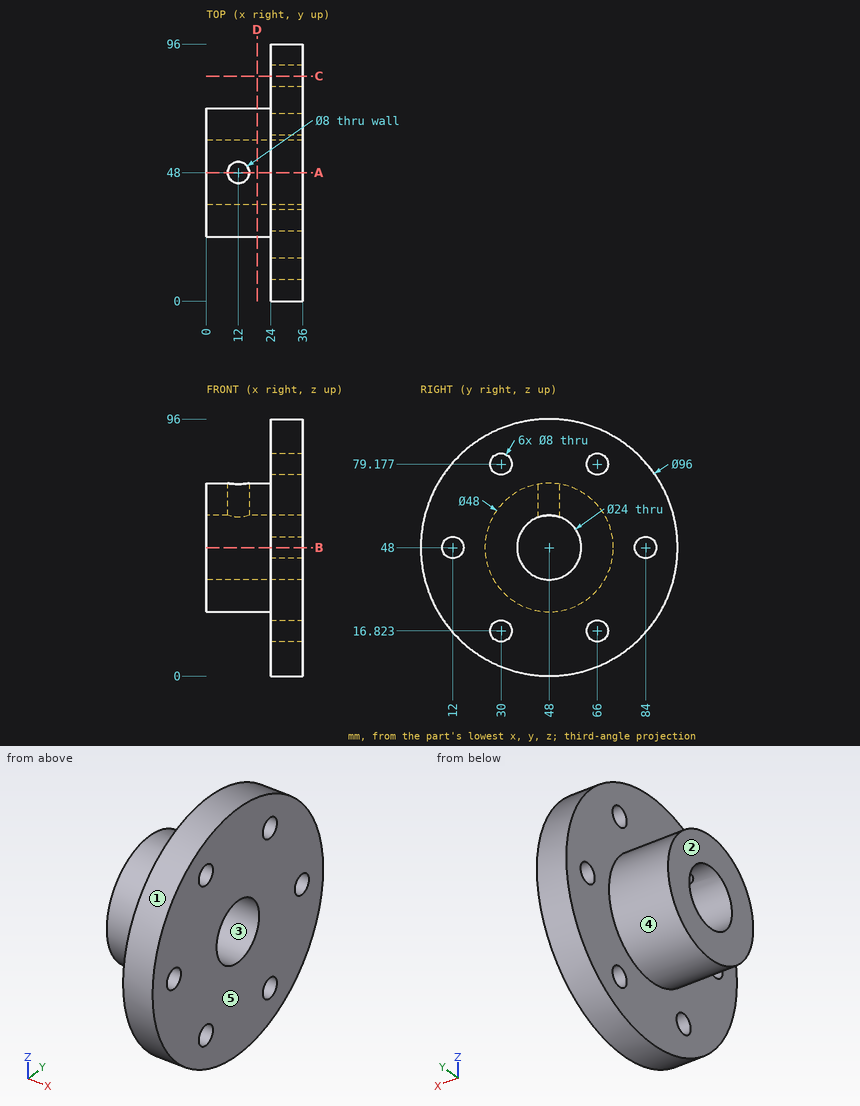
The figure shows three views and two pictorial views of one solid part (mm, origin at its lowest corner). Answer the questions. A direction names the side the tool comes from. Coordinates: 2 decimals unless noted, no trailing zeros. Loops run counter-clockwise (first coordinate to the right, second up) from the corner with the lowest first, then second, coordinate; pieces in that order, holes last. Notation, with made-up numbers: M 14.5,80 L 71.5,80 A18 ccw 71.5,115 Z; hole C 25.25,-14 d6. An arc over 180 degrees is marked long. Answer as CSV lines item,"result". Start each with the question number.
(1) For the marked faces 4 and 5, determine the directions among +Z, -Z, +X, -X, +Y, -Y from which every point of the face is accessible in a straight line to the end or side of a thin tool.
(2) The part is cut by section D-D (x = 19). Give the vertices of the cut face in (y, z), and give its area (3 significant figures).
(3) Given pin 1 (4 mm diameter, centred on x = 5.5, z = 59, fed in from -Y); pin 2 (1 mm diameter, centred on x = 12.5, z = 59, fed in from -Y); pin 3 (3 mm diameter, centred on y = 50, z = 15, fed in from -X), each flat-ended and moving along its own axis, determine where each tip first touches the part or whether it passes through.
(4) The part is cut by section B-B (z = 48). Give the vertices of the cut face in (x, y).
(5) The part is cut by section C-C (y = 84). Give the vertices of the cut face in (x, z).
(6) The mould has two halves that part along Z. Classify the marked faces 1, 2 and 3: pulls with the +Z half, pulls with the -Z half, needs draft (parallel to the pull), parting line crosses it, or undercut.
(7) The part is cut by section A-A (y = 48). Give the vertices of the cut face in (x, z).
(8) Find the intervals of material crossed by L1, parallel to X at y = 48, z = 66; L2, parallel to Z at x = 2, y = 48.5; L3, parallel to Y at x = 34.5, z = 39, in increasing order. Write a range as [from, to].
Determined:
1,face 4,"-X"
1,face 5,"+Z, -Z, +X, +Y, -Y"
2,outline,"C 48,48 d48; hole C 48,48 d24"
2,area,"1,360 mm2"
3,pin 1,"y = 25.75"
3,pin 2,"y = 26.42"
3,pin 3,"x = 24"
4,outline,"M 0,24 L 24,24 L 24,16 L 36,16 L 36,36 L 0,36 Z; M 0,60 L 36,60 L 36,80 L 24,80 L 24,72 L 0,72 Z; M 24,0 L 36,0 L 36,8 L 24,8 Z; M 24,88 L 36,88 L 36,96 L 24,96 Z"
5,outline,"M 24,16.25 L 36,16.25 L 36,44 L 24,44 Z; M 24,52 L 36,52 L 36,79.75 L 24,79.75 Z"
6,face 1,"parting line crosses it"
6,face 2,"needs draft"
6,face 3,"undercut"
7,outline,"M 0,24 L 24,24 L 24,0 L 36,0 L 36,36 L 0,36 Z; M 0,60 L 8,60 L 8,72 L 0,72 Z; M 16,60 L 36,60 L 36,96 L 24,96 L 24,72 L 16,72 Z"
8,L1,"[0, 8], [16, 36]"
8,L2,"[24.01, 36.01], [59.99, 71.99]"
8,L3,"[0.85, 40.06], [55.94, 95.15]"
